Input: part model. Units: mm. Frame: model coordinates. Face numbers are marked on the shaded views. A direction names the side the tool comes from. Round coordinates to 2 decimals unless told otherwise and drop trailing zeros. Loops run counter-clockwise (first coordinate to the right, second up) from the corner with the lowest first, then second, coordinate; pieces in that order, holes last.
(1) Cut plane A-A, the plane z = 11. Output: boundary loops of the cut face in (x, y).
(2) Cut plane C-C, the plane y = -66. Output: boundary loops of the cut face in (x, z).
(3) Line query: line 1 (Z direction, x = 14.5, y = -30); line 2 (Y direction, x = 8.5, z = 0.5); line 3 (Z direction, x = 23.25, y = 59). Output: solid intervals per line, ascending.
(4) Draft query along Z for the marked faces 3, 4 and 5. Return one class per face: released by +Z, released by -Z, zero draft, split by the parting line, or undercut.
(5) Access query for the marked faces 1 and 2. Directions: +Z, -Z, +X, -X, +Y, -Y. A direction counts if a zero-diameter tool reaches every point of the face in a straight line with its end or side. Return the directions, or none.
(6) Cut plane B-B, the plane x = 11.5. Output: boundary loops of the cut face in (y, z), and give its area (3 significant figures).
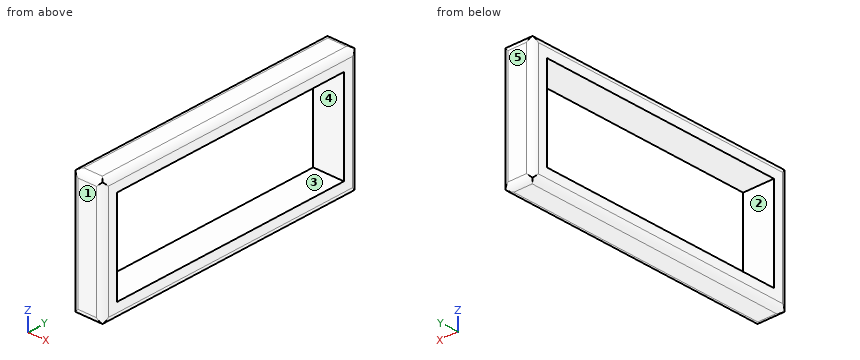
from build123d import *

# Parameters (mm, degrees)
F0_W        = 228.6
F0_H        = 101.6
F0_W_2      = 203.2
F0_H_2      = 76.2
F1_DEPTH    = 25.4
F2_R        = 5.08
F3_T1_DEPTH = 243.84
F4_T1_DEPTH = 243.84


# Not quite as in the source:
# - a fillet or chamfer that OpenCascade refuses, or shapes differently, is made with other operations: its cross-section is extruded or revolved along the edge and cut away or added


with BuildPart() as f1:
    # F0 (on Right) → F1 (new body)
    with BuildSketch(Plane.YZ):
        with Locations((0.4783831537, -17.3432382704)):
            Rectangle(F0_W, F0_H)
        with Locations((0.4783831537, -17.3432382704)):
            Rectangle(F0_W_2, F0_H_2, mode=Mode.SUBTRACT)
    extrude(amount=F1_DEPTH)

    # F2
    f2_edges = [f1.edges().sort_by_distance(p)[0] for p in [
        (12.7, -113.821617, 33.456762),
        (12.7, -113.821617, -68.143238),
        (0, -113.821617, -17.343238),
        (25.4, -113.821617, -17.343238),
        (12.7, 114.778383, -68.143238),
        (12.7, 114.778383, 33.456762),
        (0, 114.778383, -17.343238),
        (25.4, 114.778383, -17.343238),
    ]]
    fillet(f2_edges, radius=F2_R)

    # F3: fillet of radius 5.08 on 4 edges, made by hand

    # F3_s2 → F3_t1 (cut)
    with BuildSketch(Plane.XZ.offset(-122.3983831537)):
        with BuildLine():
            ThreePointArc((0, -63.0632382704), (1.4878975516, -66.6553407189), (5.08, -68.1432382704))
            Line((5.08, -68.1432382704), (0, -68.1432382704))
            Line((0, -68.1432382704), (0, -63.0632382704))
        make_face()
        with BuildLine():
            ThreePointArc((25.4, -63.0632382704), (23.9121024484, -66.6553407189), (20.32, -68.1432382704))
            Line((20.32, -68.1432382704), (25.4, -68.1432382704))
            Line((25.4, -68.1432382704), (25.4, -63.0632382704))
        make_face()
    extrude(amount=F3_T1_DEPTH, mode=Mode.SUBTRACT)

    # F4: fillet of radius 5.08 on 4 edges, made by hand

    # F4_s2 → F4_t1 (cut)
    with BuildSketch(Plane.XZ.offset(-122.3983831537)):
        with BuildLine():
            ThreePointArc((5.08, 33.4567617296), (1.4878975516, 31.968864178), (0, 28.3767617296))
            Line((0, 28.3767617296), (0, 33.4567617296))
            Line((0, 33.4567617296), (5.08, 33.4567617296))
        make_face()
        with BuildLine():
            ThreePointArc((20.32, 33.4567617296), (23.9121024484, 31.968864178), (25.4, 28.3767617296))
            Line((25.4, 28.3767617296), (25.4, 33.4567617296))
            Line((25.4, 33.4567617296), (20.32, 33.4567617296))
        make_face()
    extrude(amount=F4_T1_DEPTH, mode=Mode.SUBTRACT)


solid = f1.part
Reported:
1. outline: (0, -108.74) arc R5.08 ccw to (5.08, -113.82) - (20.32, -113.82) arc R5.08 ccw to (25.4, -108.74) - (25.4, -101.12) - (0, -101.12) - close; (0, 102.08) - (25.4, 102.08) - (25.4, 109.7) arc R5.08 ccw to (20.32, 114.78) - (5.08, 114.78) arc R5.08 ccw to (0, 109.7) - close
2. outline: (0, -63.06) arc R5.08 ccw to (5.08, -68.14) - (20.32, -68.14) arc R5.08 ccw to (25.4, -63.06) - (25.4, -55.44) - (0, -55.44) - close; (0, 20.76) - (25.4, 20.76) - (25.4, 28.38) arc R5.08 ccw to (20.32, 33.46) - (5.08, 33.46) arc R5.08 ccw to (0, 28.38) - close
3. line 1: z = -68.14 to -55.44, 20.76 to 33.46
3. line 2: y = -113.82 to -101.12, 102.08 to 114.78
3. line 3: z = -67.21 to -55.44, 20.76 to 32.53
4. face 3: undercut
4. face 4: undercut
4. face 5: zero draft
5. face 1: +Z, -Z, +X, -X, -Y
5. face 2: +X, -X
6. outline: (-113.82, -63.06) arc R5.08 ccw to (-108.74, -68.14) - (109.7, -68.14) arc R5.08 ccw to (114.78, -63.06) - (114.78, 28.38) arc R5.08 ccw to (109.7, 33.46) - (-108.74, 33.46) arc R5.08 ccw to (-113.82, 28.38) - close; hole (-101.12, -55.44) - (102.08, -55.44) - (102.08, 20.76) - (-101.12, 20.76) - close
6. area: 7,720 mm2
